```python
from build123d import *

# Parameters (mm, degrees)
BOSS_EXTRUDE1_DEPTH         = 240
SKETCH5_R                   = 136
BOSS_EXTRUDE2_DEPTH         = 30
IZIM1_R                     = 23.5
KES_EKSTR_ZYON1_DEPTH       = 80
IZIM2_R                     = 25
IZIM2_R_2                   = 10
Y_KSEKLIK_EKSTR_ZYON1_DEPTH = 10
SCALE1_SCALE                = 0.25
SKETCH6_R                   = 6
CUT_EXTRUDE1_DEPTH          = 200


with BuildPart() as part:
    # Sketch1 → Boss-Extrude1 (new body)
    with BuildSketch(Plane(origin=(0, 0, 0), x_dir=(1, 0, 0), z_dir=(0, 1, 0))):
        Polygon((0, -20), (0, -6), (290, -6), (290, -134), (0, -134), (0, -120), (260, -120), (260, -20), align=None)
    extrude(amount=BOSS_EXTRUDE1_DEPTH)

    # Sketch5 → Boss-Extrude2 (add)
    with BuildSketch(Plane(origin=(290, 0, 0), x_dir=(0, 0, -1), z_dir=(1, 0, 0))):
        with Locations((-60, 120)):
            Circle(SKETCH5_R)
    extrude(amount=BOSS_EXTRUDE2_DEPTH)

    # Çizim1 → Kes-Ekstrüzyon1 (cut)
    with BuildSketch(Plane(origin=(320, 0, 0), x_dir=(0, 0, -1), z_dir=(1, 0, 0))):
        with Locations((-60, 120)):
            Circle(IZIM1_R)
    extrude(amount=-KES_EKSTR_ZYON1_DEPTH, mode=Mode.SUBTRACT)

    # Çizim2 → Yükseklik-Ekstrüzyon1 (add)
    with BuildSketch(Plane.ZY.offset(-260)):
        with Locations((60, 120)):
            Circle(IZIM2_R)
        with Locations((60, 120)):
            Circle(IZIM2_R_2, mode=Mode.SUBTRACT)
    extrude(amount=-Y_KSEKLIK_EKSTR_ZYON1_DEPTH)


with BuildPart() as part_1:
    # Scale1: scaled about (228.089824151, 120, 66.174750275)
    add(part.part.scale(SCALE1_SCALE).moved(Location((171.067368113, 90, 49.631062706))))

    # Sketch6 → Cut-Extrude1 (cut)
    with BuildSketch(Plane.XY.offset(83.131062707)):
        with Locations((186.067368113, 120)):
            Circle(SKETCH6_R)
    extrude(amount=-CUT_EXTRUDE1_DEPTH, mode=Mode.SUBTRACT)


solid = part_1.part
```
Verification items for the finished model (mm, model axes). A direction names the side the tool comes from. Round coordinates to 2 decimals unless told otherwise and drop trailing zeros. Order: outer loops, then holes, each group sorted by start corner. A loop starts at its lowest first (then second) coordinate and runs counter-clockwise, first axis right, second up. Notation, with made-up numbers: (43.5, 17.5) - (76.5, 17.5) arc R29 cw to (76.5, 55.5) - close; hole circle Ø2 at (-13.75, -16.5). An arc over 180 degrees is marked (long way). Use CSV: the item, a comma, the result in double quotes. Start each with the question number.
1) Section check B-B, the plane x = 196. Record the cut outline in (y, z).
2) Access from +Z, -Z, +X, -X, +Y, -Y to the whole of each face (thin tool, end or side, straight path). Record for faces 4 (the flat face through (238.567, 117, 65)), 5 (the flat face through (243.567, 120, 89)), 6 (the flat face through (204, 120, 54.631)), 7 (the flat face through (207, 120, 51.131)).
3) Section check C-C, the plane z = 64. Record the cut outline in (x, y).
4) Go/stop test with flat-tipped pins: P1, Ø10, axis at x = 199, z = 57.5, coming from the -Y side; P2, Ø1.5, axis at x = 240, y = 129, coming from the +Z side; P3, Ø15.5, axis at x = 186.07, y = 120, coming from the -Z side. Record where each tip stops, or that it passes through.
5) Thickness scan on L1, parallel to Z at x = 192.5, y = 140; L2, parallel to X at y = 123, z = 74; L3, parallel to X at y = 140.5, z = 40.5. Record the ranges inside material, lowest first.
6) Section check A-A, the plane y = 120. Record the cut outline in (x, z).
7) Mould release check, pull along Y, two halves, no side actions. Record for faces 1 (the cylindrical face through (237.3, 122.108, 65.975)), 2 (the flat face through (218, 90, 54)), 3 (the flat face through (203, 120, 79.631)): +Y half, -Y half, draft (parallel to the pull), parting line (faces both ways), or undercut.
8) Section check D-D, the plane x = 185.5. Record the cut outline in (y, z), plus the area to 3 significant figures.
Answers:
1,outline,"(90, 51.13) - (150, 51.13) - (150, 54.63) - (90, 54.63) - close; (90, 79.63) - (150, 79.63) - (150, 83.13) - (90, 83.13) - close"
2,face 4,"+X"
2,face 5,"+Z, -X, +Y, -Y"
2,face 6,"-X, +Y, -Y"
2,face 7,"-Z, -X, +Y, -Y"
3,outline,"(236.07, 90) - (243.57, 90) - (243.57, 86.01) - (251.07, 86.01) - (251.07, 114.16) - (238.57, 114.16) - (238.57, 117.58) - (236.07, 117.58) - close; (236.07, 122.42) - (238.57, 122.42) - (238.57, 125.84) - (251.07, 125.84) - (251.07, 153.99) - (243.57, 153.99) - (243.57, 150) - (236.07, 150) - close"
4,P1,"stops at y = 90"
4,P2,"stops at z = 83.13"
4,P3,"stops at z = 51.13"
5,L1,"z = 51.13 to 54.63, 79.63 to 83.13"
5,L2,"x = 236.07 to 251.07"
5,L3,"x = 243.57 to 251.07"
6,outline,"(171.07, 51.13) - (180.07, 51.13) - (180.07, 54.63) - (171.07, 54.63) - close; (171.07, 79.63) - (180.07, 79.63) - (180.07, 83.13) - (171.07, 83.13) - close; (192.07, 51.13) - (243.57, 51.13) - (243.57, 30.63) - (251.07, 30.63) - (251.07, 58.76) - (238.57, 58.76) - (238.57, 62.13) - (236.07, 62.13) - (236.07, 54.63) - (192.07, 54.63) - close; (192.07, 79.63) - (236.07, 79.63) - (236.07, 67.13) - (238.57, 67.13) - (238.57, 70.51) - (251.07, 70.51) - (251.07, 98.63) - (243.57, 98.63) - (243.57, 83.13) - (192.07, 83.13) - close"
7,face 1,"undercut"
7,face 2,"-Y half"
7,face 3,"draft"
8,outline,"(90, 51.13) - (114.03, 51.13) - (114.03, 54.63) - (90, 54.63) - close; (90, 79.63) - (114.03, 79.63) - (114.03, 83.13) - (90, 83.13) - close; (125.97, 51.13) - (150, 51.13) - (150, 54.63) - (125.97, 54.63) - close; (125.97, 79.63) - (150, 79.63) - (150, 83.13) - (125.97, 83.13) - close"
8,area,"336 mm²"
